Autodesk Fusion 360 part; units mm, degrees
sketch "Sketch1" plane through (0, 0, 0) normal (0, 1, 0) x (1, 0, 0)
  line L0 (-0.0152, -15) -> (0.0152, -15)
  line L1 (0.0062, 15) -> (-0.0062, 15)
  line L2 (0, 15) -> (0, -15) construction
  line L3 (-7.1875, 7.5003) -> (-6.5096, -8.7706)
  line L4 (7.1875, 7.5003) -> (6.5096, -8.7706)
  arc A0 (0.0062, 15) -> (-7.1875, 7.5003) centre (0.0062, 7.8) ccw
  arc A1 (7.1875, 7.5003) -> (-0.0062, 15) centre (-0.0062, 7.8) ccw
  arc A2 (-6.5096, -8.7706) -> (-0.0152, -15) centre (-0.0152, -8.5) ccw
  arc A3 (0.0152, -15) -> (6.5096, -8.7706) centre (0.0152, -8.5) ccw
  point P0 (-6.25, -15)
  point P1 (6.25, -15)
  point P2 (-7.5, 15)
  point P3 (7.5, 15)
  dimension "d1" = 12.5
  dimension "d2" = 15
  dimension "d3" = 30
  dimension "d4" = 15
  dimension "d6" = 7.2
  dimension "d7" = 6.5
extrude "Extrude1" add sketch "Sketch1" along normal blind 5
sketch "Sketch2" plane through (0, 5, 0) normal (0, 1, 0) x (-1, 0, 0)
  arc A0 (-7.1875, -7.5003) -> (0, -15) centre (0.0062, -7.8) ccw
  arc A1 (0, -15) -> (7.1875, -7.5003) centre (-0.0062, -7.8) ccw
  line L0 (7.1875, -7.5003) -> (6.5096, 8.7706)
  arc A2 (6.5096, 8.7706) -> (0.0152, 15) centre (0.0152, 8.5) ccw
  line L1 (0.0152, 15) -> (-0.0152, 15)
  arc A3 (-0.0152, 15) -> (-6.5096, 8.7706) centre (-0.0152, 8.5) ccw
  line L2 (-6.5096, 8.7706) -> (-7.1875, -7.5003)
  line L3 (-0.0152, 15) -> (-0.0152, 10) construction
  circle A4 centre (-0.0152, 10) radius 2
  dimension "d10" = 5
  dimension "d11" = 4
extrude "Extrude2" cut sketch "Sketch2" against normal blind 7 contours A4
The listing builds one solid part. Answer for the finished solid, in the listing's coordinates (mm). Coordinates: 2 decimals unless noted, no trailing zeros. Loops run counter-clockwise (first coordinate to the right, second up) from the corner with the lowest first, then second, coordinate; pieces in that order, holes last. Notation, with made-up numbers: (18, -18.5) -> (50, -18.5) arc R21 cw to (50, 5.5) -> close; hole circle Ø6 at (40, -39). An arc over 180 degrees is marked (long way). Answer in a Markdown table with one row per item. Add a question column.
1. Determine the mould class of faces 1 (the cylindrical face through (-4.464, 2.465, 13.239)), 2 (the flat face through (0, 5, 0)), 3 (the cylindrical face through (0, 3, 12)) for opening direction Z: +Z half, -Z half, draft (parallel to the pull), parting line (faces both ways), or undercut.
2. Consider line 1 (X direction, y = 1.45, z = 9.5); line 2 (X direction, y = 4.5, z = -1.75); line 3 (Z direction, x = 3, y = 0.8). Determine where each line is inside the solid, lowest interval first. Write a range as [from, to].
3. The part is cut by section A-A, the plane x = -1. Write down the section's boundary in (y, z), then the cut area to 3 significant figures.
4. The part is cut by section D-D, the plane z = -4. Write down the section's boundary in (x, y), then the cut area to 3 significant figures.
5. The part is cut by section B-B, the plane z = 10. Write down the section's boundary in (x, y), then the cut area to 3 significant figures.
6. Flat-ended cylindrical pins translate along their axes: P1, Ø3.5, axis at x = 0.02, z = 10, coming from the -Y side; P2, Ø1, axis at x = -3.5, y = 2, coming from the -Z side. Find the tip coordinate at first contact, or state that the pin passes through.
Answer below:
| question | item | result |
|---|---|---|
| 1 | face 1 | +Z half |
| 1 | face 2 | draft |
| 1 | face 3 | undercut |
| 2 | line 1 | [-6.44, -1.92], [1.95, 6.44] |
| 2 | line 2 | [-6.95, 6.95] |
| 2 | line 3 | [-14.34, 14.27] |
| 3 | outline | (0, -14.93) -> (5, -14.93) -> (5, 8.28) -> (0, 8.28) -> close; (0, 11.72) -> (5, 11.72) -> (5, 14.92) -> (0, 14.92) -> close |
| 3 | area | 132 mm2 |
| 4 | outline | (-7.04, 0) -> (7.04, 0) -> (7.04, 5) -> (-7.04, 5) -> close |
| 4 | area | 70.4 mm2 |
| 5 | outline | (-6.34, 0) -> (-1.98, 0) -> (-1.98, 5) -> (-6.34, 5) -> close; (2.02, 0) -> (6.34, 0) -> (6.34, 5) -> (2.02, 5) -> close |
| 5 | area | 43.4 mm2 |
| 6 | P1 | through |
| 6 | P2 | z = -14.34 |
